Input: dimensioned drawing with shaded views. Units: mm. Origin: part minimum x, y, z. Round coordinates to 2 decimals unless told otherwise and drop trailing zeros. Loops run counter-clockwise (first coordinate to the right, second up) from the corner with the lowest first, then second, coordinate; pieces in that order, holes last. Notation, with made-up numbers: (19.25, 19.5) - (32.25, 19.5) arc R33 cw to (32.25, 47.5) - close; hole circle Ø7 at (69.25, -38). An arc over 180 degrees is marked (long way). Use CSV: the item, a comma, the result in double quotes. Start each with the question number.
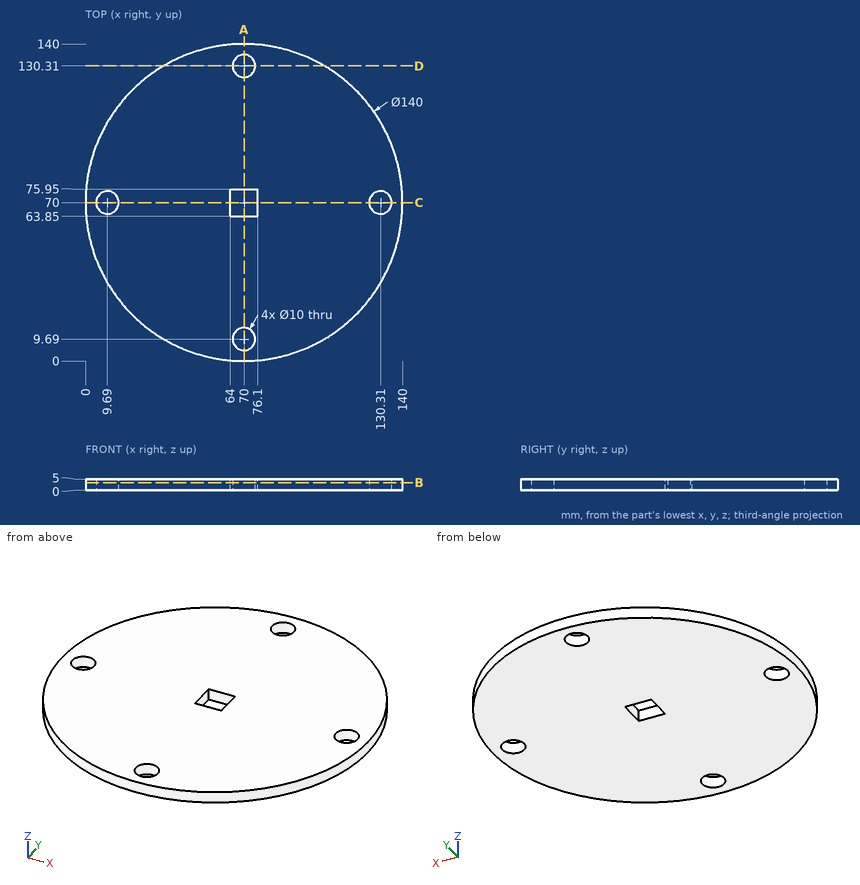
1. Section query D-D on y = 130.31. Return the cut outline in (x, z).
2. Line query: line 1 along Y through (x, z) = (70, 3.55); line 2 along Y through (x, z) = (9.69, 3.95); line 3 along Y through (x, z) = (9.5, 4.6). Output: solid intervals per line, ascending.
3. Section query C-C on y = 70. Return the cut outline in (x, z).
4. Section query B-B on z = 3.4. Return the cut outline in (x, y).
5. Section query A-A on x = 70. Return the cut outline in (y, z).
6. Contact query for a flat-ended pin moving along its axis: P1, Ø2.5, axis at y = 72.5, z = 2.5, coming from the +X side. Output: stop coordinate, or through.
Values:
1,outline,"(34.47, 0) - (65, 0) - (65, 5) - (34.47, 5) - close; (75, 0) - (105.53, 0) - (105.53, 5) - (75, 5) - close"
2,line 1,"y = 0 to 4.69, 14.69 to 63.85, 75.95 to 125.31, 135.31 to 140"
2,line 2,"y = 34.47 to 65, 75 to 105.53"
2,line 3,"y = 34.79 to 65, 75 to 105.21"
3,outline,"(0, 0) - (4.69, 0) - (4.69, 5) - (0, 5) - close; (14.69, 0) - (64, 0) - (64, 5) - (14.69, 5) - close; (76.1, 0) - (125.31, 0) - (125.31, 5) - (76.1, 5) - close; (135.31, 0) - (140, 0) - (140, 5) - (135.31, 5) - close"
4,outline,"circle Ø140 at (70, 70); hole circle Ø10 at (9.69, 70); hole (64, 63.85) - (76.1, 63.85) - (76.1, 75.95) - (64, 75.95) - close; hole circle Ø10 at (70, 9.69); hole circle Ø10 at (70, 130.31); hole circle Ø10 at (130.31, 70)"
5,outline,"(0, 0) - (4.69, 0) - (4.69, 5) - (0, 5) - close; (14.69, 0) - (63.85, 0) - (63.85, 5) - (14.69, 5) - close; (75.95, 0) - (125.31, 0) - (125.31, 5) - (75.95, 5) - close; (135.31, 0) - (140, 0) - (140, 5) - (135.31, 5) - close"
6,P1,"stops at x = 139.99"
